Work out the finished part from the listing and answer in its coordinate system (mm). Coordinates: 2 decimals unless noted, no trailing zeros. Loops run counter-clockwise (first coordinate to the right, second up) from the corner with the lowest first, then second, coordinate; pieces in that order, holes last. Notation, with made-up numbers: (7, -13) - (30, -13) arc R9 cw to (30, 0) - close; hole circle Ø11 at (-4, -11.5). An arc over 180 degrees is marked (long way). Write each question's results on one line, items separated by ' | '. Start each with the question number.
1. A cutting plane is placed at A-A on y = -494.5. Determine the outline of the cut face in (x, z).
2. A cutting plane is placed at C-C on z = 3.55. Determine the outline of the cut face in (x, y), then the cut area to 3 significant figures.
3. Find the intervals of material crossed by line 1 along Y through (x, z) = (25, 1.65); line 2 along Y through (x, z) = (16, 2.55); line 3 along Y through (x, z) = (40.5, 2.75), in increasing order. Write a range as [from, to].
4. A cutting plane is placed at B-B on x = 26. Determine the outline of the cut face in (y, z), then the cut area to 3 significant figures.
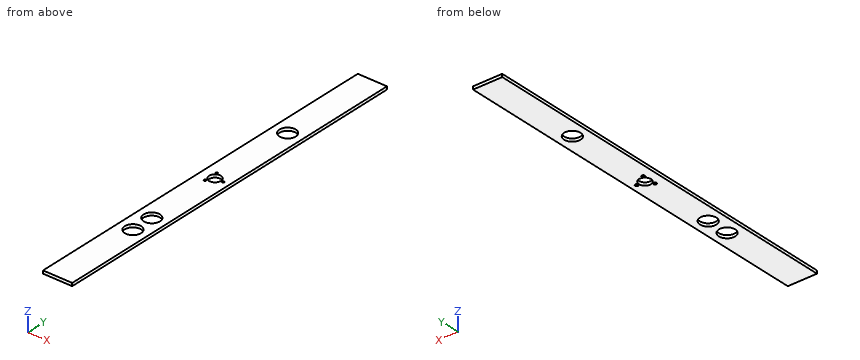
from build123d import *

# Parameters (mm, degrees)
ESQUISSE1_W        = 50
ESQUISSE1_H        = 650
ESQUISSE1_R        = 10.25
ESQUISSE1_R_2      = 14
ESQUISSE1_R_3      = 1.75
BOSS_EXTRU_1_DEPTH = 5
CHANFREIN1_SIZE    = 1


with BuildPart() as part:
    # Esquisse1 → Boss.-Extru.1 (new body)
    with BuildSketch(Plane.XY):
        with Locations((25, -325)):
            Rectangle(ESQUISSE1_W, ESQUISSE1_H)
        with Locations((25, -325)):
            Circle(ESQUISSE1_R, mode=Mode.SUBTRACT)
        with Locations((25, -494.5)):
            Circle(ESQUISSE1_R_2, mode=Mode.SUBTRACT)
        with Locations((18, -312.875644347)):
            Circle(ESQUISSE1_R_3, mode=Mode.SUBTRACT)
        with Locations((18, -337.124355653)):
            Circle(ESQUISSE1_R_3, mode=Mode.SUBTRACT)
        with Locations((39, -325)):
            Circle(ESQUISSE1_R_3, mode=Mode.SUBTRACT)
        with Locations((25, -455.5)):
            Circle(ESQUISSE1_R_2, mode=Mode.SUBTRACT)
        with Locations((25, -175)):
            Circle(ESQUISSE1_R_2, mode=Mode.SUBTRACT)
    extrude(amount=BOSS_EXTRU_1_DEPTH)

    # Chanfrein1
    chanfrein1_edges = [part.edges().sort_by_distance(p)[0] for p in [
        (16.25, -312.875644347, 0),
        (37.25, -325, 0),
        (16.25, -337.124355653, 0),
    ]]
    chamfer(chanfrein1_edges, length=CHANFREIN1_SIZE)


solid = part.part
Values:
1) outline: (0, 0) - (11, 0) - (11, 5) - (0, 5) - close; (39, 0) - (50, 0) - (50, 5) - (39, 5) - close
2) outline: (0, -650) - (50, -650) - (50, 0) - (0, 0) - close; hole circle Ø28 at (25, -494.5); hole circle Ø28 at (25, -455.5); hole circle Ø28 at (25, -175); hole circle Ø20.5 at (25, -325); hole circle Ø3.5 at (18, -337.12); hole circle Ø3.5 at (18, -312.88); hole circle Ø3.5 at (39, -325) | area: 30,300 mm^2
3) line 1: [-650, -508.5], [-480.5, -469.5], [-441.5, -335.25], [-314.75, -189], [-161, 0] | line 2: [-650, -505.22], [-483.78, -466.22], [-444.78, -329.91], [-320.09, -185.72], [-164.28, 0] | line 3: [-650, -325.9], [-324.1, 0]
4) outline: (-650, 0) - (-508.46, 0) - (-508.46, 5) - (-650, 5) - close; (-480.54, 0) - (-469.46, 0) - (-469.46, 5) - (-480.54, 5) - close; (-441.54, 0) - (-335.2, 0) - (-335.2, 5) - (-441.54, 5) - close; (-314.8, 0) - (-188.96, 0) - (-188.96, 5) - (-314.8, 5) - close; (-161.04, 0) - (0, 0) - (0, 5) - (-161.04, 5) - close | area: 2,730 mm^2
